Job drawing, mm, ordinate dimensions from the low corner. One solid piece. Give positions to 0.01 mm unless a question says otherwise; leave off trailing zeros. Write each loop counter-clockwise with the first axis right and the second up, starting at its lowest first coordinate (ties: lowest second). Pieces come first, ordered by that corner, then holes. Notation, with made-up numbers: (56, 0) - (105, 0) arc R21 cw to (105, 11) - close; hole circle Ø4 at (13.5, 68). An arc over 180 degrees is marked (long way). Answer in a Markdown table with one row per item. Add a question column.
1. Band-saw the part on A-A on x = 26. Write the cut outline in (y, z).
2. Band-saw the part on D-D on x = 37. Write the cut outline in (y, z), plus the area to 3 significant figures.
3. Probe line 1 along Z through (x, y) = (26, 1.05); line 2 along Z through (x, y) = (9.5, 2.2) (1 decimal); line 3 along X through (y, z) = (2.05, 57.5). List the from-to ranges inside material, lowest first.
4. Drop flat-ended pins along their axis: pin 1 Ø1.5 at (x, z) = (35.5, 24) entering from -Y; pin 2 Ø1.5 at (x, y) = (37, 2) entering from +Z (1 decimal); pin 3 Ø1 at (x, y) = (21, 0.5) entering from +Z; pin 4 Ø6 at (x, z) = (39.5, 50.5) entering from -Y. Give the stop position or say it passes through.
5. Band-saw the part on B-B on z = 10. Write the cut outline in (x, y), plus the area to 3 significant figures.
6. Band-saw the part on C-C on z = 48.5. Write the cut outline in (x, y).
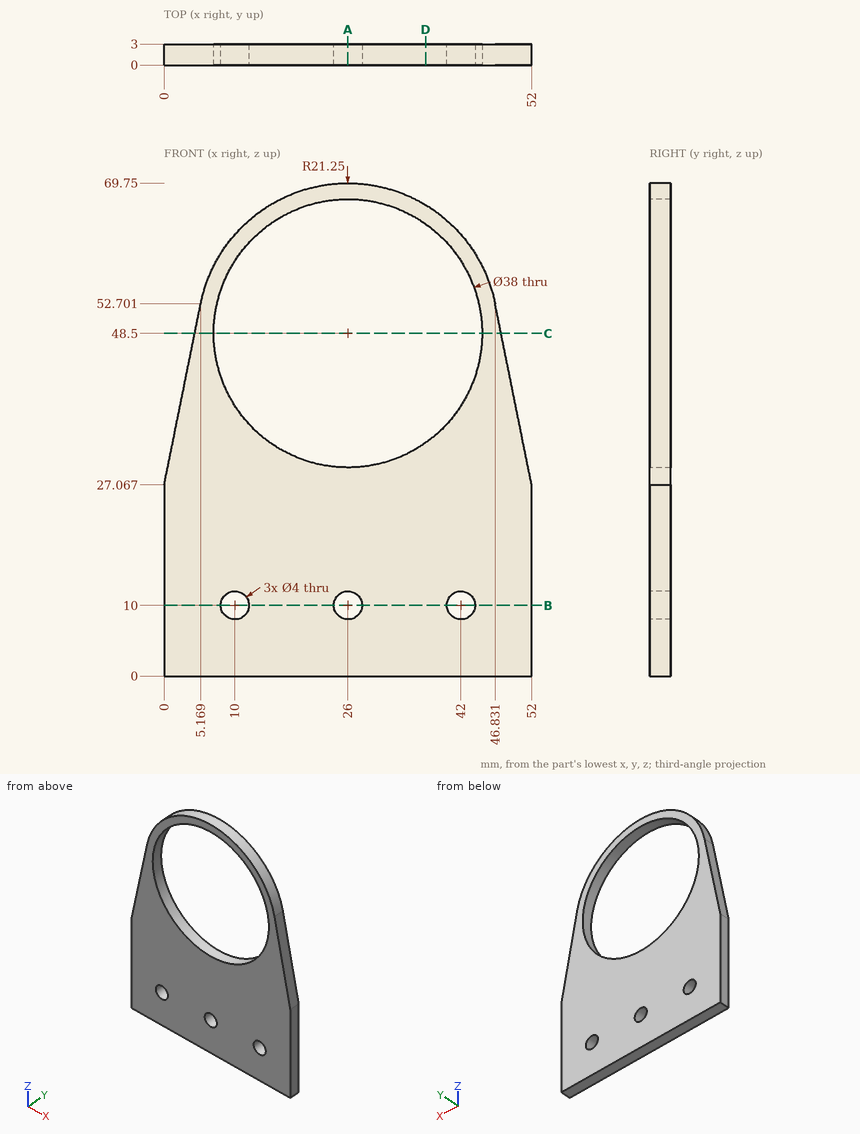
Values:
| question | item | result |
|---|---|---|
| 1 | outline | (0, 0) - (3, 0) - (3, 8) - (0, 8) - close; (0, 12) - (3, 12) - (3, 29.5) - (0, 29.5) - close; (0, 67.5) - (3, 67.5) - (3, 69.75) - (0, 69.75) - close |
| 2 | outline | (0, 0) - (3, 0) - (3, 33.01) - (0, 33.01) - close; (0, 63.99) - (3, 63.99) - (3, 66.68) - (0, 66.68) - close |
| 2 | area | 107 mm² |
| 3 | line 1 | z = 0 to 8, 12 to 29.5, 67.5 to 69.75 |
| 3 | line 2 | z = 0 to 8.1, 11.9 to 39.1, 57.9 to 61.9 |
| 3 | line 3 | x = 6.75 to 9.27, 42.73 to 45.25 |
| 4 | pin 1 | stops at y = 0 |
| 4 | pin 2 | stops at z = 67.1 |
| 4 | pin 3 | stops at z = 69.27 |
| 4 | pin 4 | passes through |
| 5 | outline | (0, 0) - (8, 0) - (8, 3) - (0, 3) - close; (12, 0) - (24, 0) - (24, 3) - (12, 3) - close; (28, 0) - (40, 0) - (40, 3) - (28, 3) - close; (44, 0) - (52, 0) - (52, 3) - (44, 3) - close |
| 5 | area | 120 mm² |
| 6 | outline | (4.32, 0) - (7, 0) - (7, 3) - (4.32, 3) - close; (45, 0) - (47.68, 0) - (47.68, 3) - (45, 3) - close |
